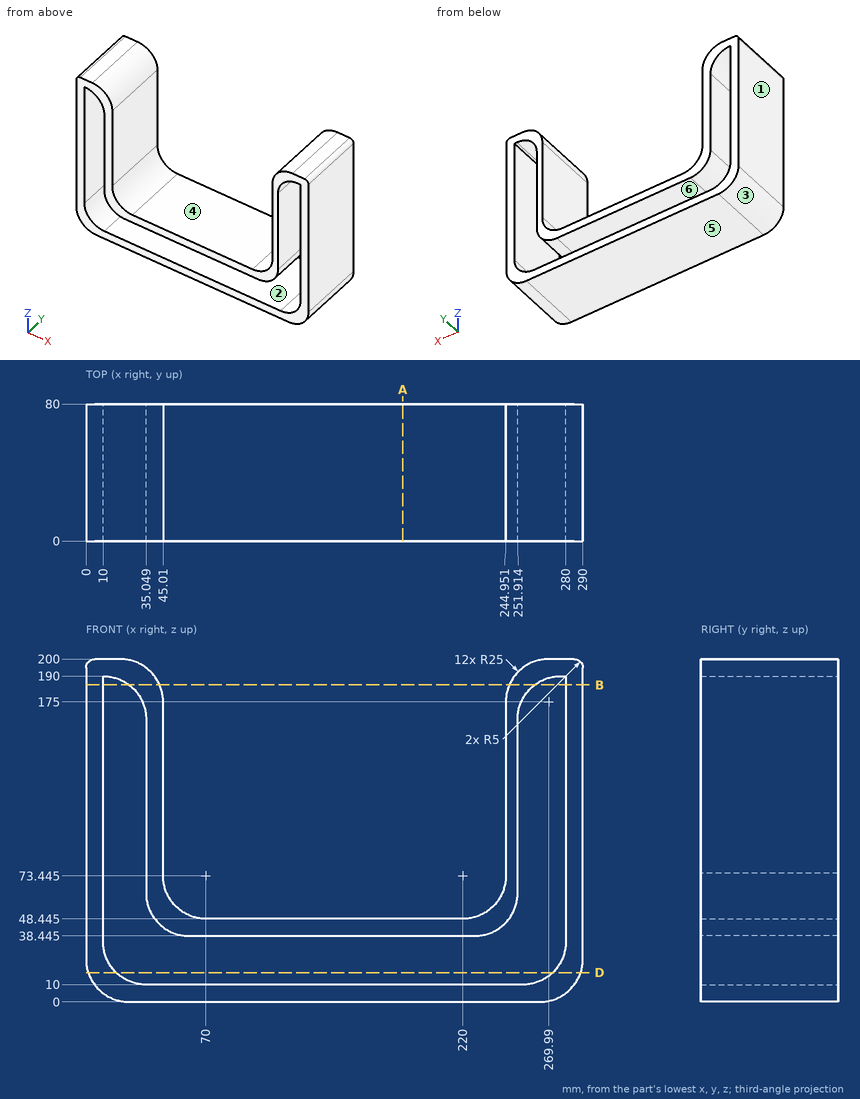
Study the drawing (mm; zero at the part's minimum x, y, z) and answer. A direction names the side the tool comes from. Round coordinates to 2 decimals unless told otherwise and drop trailing zeros. Write each loop counter-clockwise with the first axis right and the second up, starting at its lowest first coordinate (ties: lowest second). Pieces come first, ordered by that corner, then holes. Notation, with made-up numbers: (8, 4) -> (13, 4) arc R21 ccw to (13, 27) -> close; hole circle Ø9 at (72, 67.25). An arc over 180 degrees is marked (long way). Write item = value, one per line.
1) Section D-D on z = 17 is taken. Write down the section's boundary in (x, y).
Check values:
outline = (1.31, 0) -> (17.65, 0) -> (17.65, 80) -> (1.31, 80) -> close; (272.35, 0) -> (288.69, 0) -> (288.69, 80) -> (272.35, 80) -> close
2) Given pin 1 (0.9 mm diameter, centred on x = 278.5, y = 33.5, fed in from -Z); pin 2 (1.5 mm diameter, centred on x = 52.5, y = 37.5, fed in from +Z); pin 3 (3 mm diameter, centred on y = 56.5, z = 20, fed in from +X), each flat-ended and moving along its own axis, determine where each tip first touches the part or whether it passes through.
Check values:
pin_1 = 3.68
pin_2 = 56.36
pin_3 = 289.75
3) Which of the six approach directions +Z, -Z, +X, -X, +Y, -Y give full straight-line access (tool end or side, diameter ignored) to the marked faces 4, 5 and 6?
Check values:
face_4 = +Z, +Y, -Y
face_5 = -Z, +X, -X, +Y, -Y
face_6 = +Y, -Y
4) Section A-A on x = 185 is taken. Write down the section's boundary in (y, z) (1 decimal).
Check values:
outline = (0, 0) -> (80, 0) -> (80, 10) -> (0, 10) -> close; (0, 38.4) -> (80, 38.4) -> (80, 48.4) -> (0, 48.4) -> close
5) For a pull along Z with two mould halves and no side action, classify the marked faces 1, 2 and 3 as released by +Z, released by -Z, zero draft, split by the parting line, or undercut.
Check values:
face_1 = zero draft
face_2 = undercut
face_3 = released by -Z
6) Straight lines are drawn through the part: line 1 along X through (y, z) = (16, 124); line 2 along Z through (x, y) = (177, 64) (1 decimal); line 3 along X through (y, z) = (60.5, 61). For each, find the intervals that lie inside material, in ascending order. Write a range as [from, to].
Check values:
line_1 = [0, 10], [35.05, 45.03], [244.97, 251.91], [280, 290]
line_2 = [0, 10], [38.4, 48.4]
line_3 = [0, 10], [35.17, 48.32], [241.68, 251.79], [280, 290]
7) Section B-B on z = 185 is taken. Write down the section's boundary in (x, y).
Check values:
outline = (0, 0) -> (10, 0) -> (10, 80) -> (0, 80) -> close; (25.05, 0) -> (42.92, 0) -> (42.92, 80) -> (25.05, 80) -> close; (247.08, 0) -> (261.91, 0) -> (261.91, 80) -> (247.08, 80) -> close; (280, 0) -> (290, 0) -> (290, 80) -> (280, 80) -> close
